Source: three-view drawing plus pictorial views. Frame: mm from the lowest corner of the part. Round coordinates to 2 decimals unless told otherwise and drop trailing zeros. Write each loop counter-clockwise with the first axis right and the second up, starting at its lowest first coordinate (ties: lowest second). Pieces come first, ordered by that corner, then holes. Notation, with made-up numbers: (-8.5, -37) -> (24.5, -37) arc R13 ccw to (24.5, -20) -> close; hole circle Ø7 at (-7, 33.25). An arc over 180 degrees is marked (long way). Put each result on its own line as item: value.
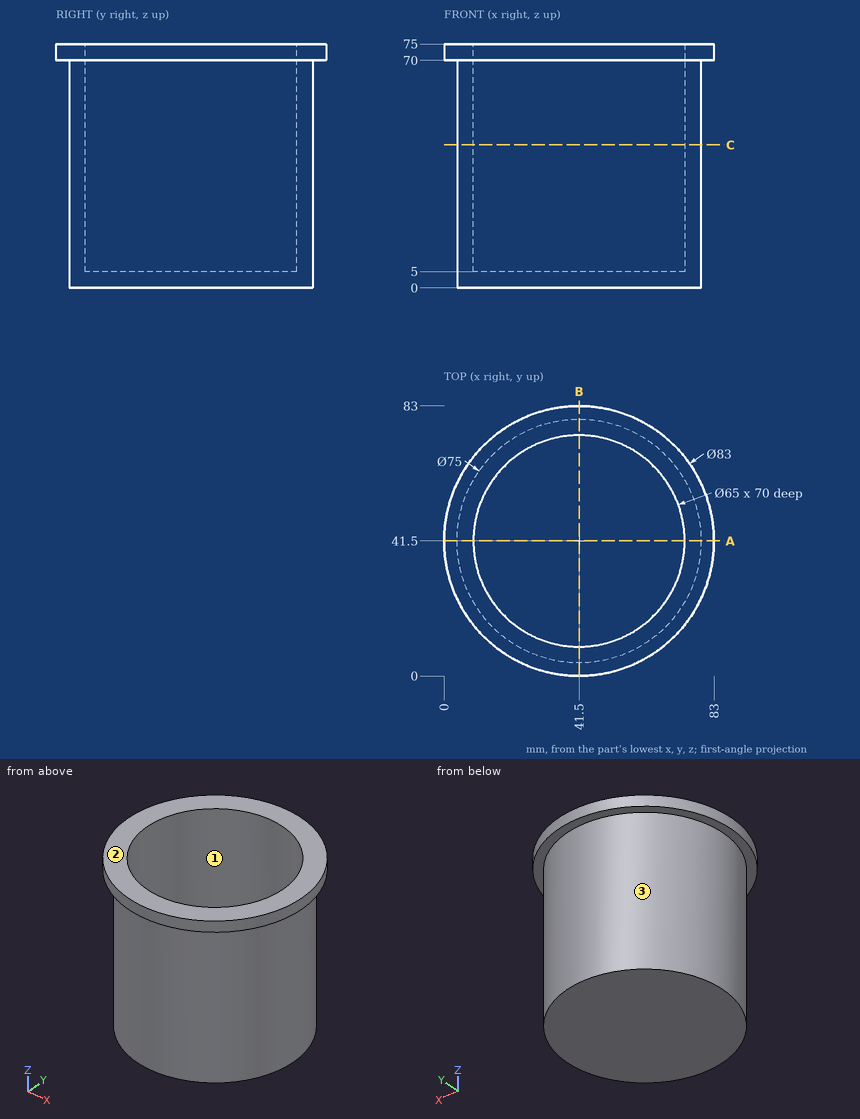
Q1. Pin query (flat end, axial travel): pin 1 (8 mm diameter, centred on x = 22, z = 15, fed in from +Y); pin 2 (2 mm diameter, centred on y = 12.5, z = 46.5, fed in from -X); pin 3 (1 mm diameter, centred on x = 60.5, z = 44.5, fed in from +Y). Return the tip coordinate at first contact, or that it passes through.
Ans:
pin 1: stops at y = 75.65
pin 2: stops at x = 16.56
pin 3: stops at y = 74.12
Q2. Draft query along Y for the marked faces 1, 2 and 3. Return one class per face: +Y half, -Y half, draft (parallel to the pull), parting line (faces both ways), or undercut.
Ans:
face 1: undercut
face 2: draft
face 3: parting line
Q3. Cut plane A-A on y = 41.5. Output: boundary loops of the cut face in (x, z), and give its area (4 significant figures).
Ans:
outline: (0, 70) -> (4, 70) -> (4, 0) -> (79, 0) -> (79, 70) -> (83, 70) -> (83, 75) -> (74, 75) -> (74, 5) -> (9, 5) -> (9, 75) -> (0, 75) -> close
area: 1,115 mm^2
Q4. Cut plane C-C on z = 44. Output: boundary loops of the cut face in (x, y), and give its area (3 significant figures).
Ans:
outline: circle Ø75 at (41.5, 41.5); hole circle Ø65 at (41.5, 41.5)
area: 1,100 mm^2
Q5. Material intervals for line 1 (X direction, y = 41, z = 49); line 2 (X direction, y = 29, z = 39.5), sorted ascending. Write a range as [from, to].
Ans:
line 1: x = [4, 9], [74, 79]
line 2: x = [6.14, 11.5], [71.5, 76.86]
